```python
from build123d import *

# Parameters (mm, degrees)
EXTRUDE_1_DEPTH     = 3
SKETCH_3_R          = 7
CUT_EXTRUDE_1_DEPTH = 65.474801279
SKETCH_4_R          = 1
CUT_EXTRUDE_2_DEPTH = 65.474801279
FILLET_1_RADIUS     = 6
FILLET_1_LENGTH     = 3
EXTRUDE_2_DEPTH     = 2
SKETCH_7_R          = 4
CUT_EXTRUDE_3_DEPTH = 65.598761598
CUT_EXTRUDE_4_DEPTH = 2
SKETCH_9_R          = 0.537141257
CUT_EXTRUDE_5_DEPTH = 65.474801279
SKETCH_10_R         = 1.85
CUT_EXTRUDE_6_DEPTH = 1.5


with BuildPart() as part:
    # 草图1 → 凸台-拉伸1 (new body)
    with BuildSketch(Plane.XY):
        Polygon((-18, 0), (18, 0), (18, 5), (-12.599564267, 58), (-28, 58), (-28, 46), (-18, 46), align=None)
    extrude(amount=EXTRUDE_1_DEPTH)

    # 草图3 → 切除-拉伸1 (cut, through all)
    with BuildSketch(Plane.XY.offset(3)):
        with Locations((-6.476357534, 13.687539211)):
            Circle(SKETCH_3_R)
    extrude(amount=-CUT_EXTRUDE_1_DEPTH, mode=Mode.SUBTRACT)

    # 草图4 → 切除-拉伸2 (cut, through all)
    with BuildSketch(Plane.XY.offset(3)):
        with Locations((12, 2.5)):
            Circle(SKETCH_4_R)
        with Locations(Location((-12, 2.5, 0), (0, 0, 180))):
            Circle(SKETCH_4_R)
    extrude(amount=-CUT_EXTRUDE_2_DEPTH, mode=Mode.SUBTRACT)

    # 圆角1: full round fillet: the end face becomes a half cylinder, R = half its width
    fillet_1_face = Plane((-28, 52, 1.5), x_dir=(0, 0, 1), z_dir=(-1, 0, 0))  # on the end face: x along it, z out of the body
    fillet_1_slab = fillet_1_face.offset(-FILLET_1_RADIUS / 2) * Box(FILLET_1_LENGTH, 2 * FILLET_1_RADIUS, FILLET_1_RADIUS, mode=Mode.PRIVATE)  # the body's end, R deep
    fillet_1_round = Plane((-22, 52, 1.5), x_dir=(-1, 0, 0), z_dir=(0, 0, 1)) * Cylinder(FILLET_1_RADIUS, FILLET_1_LENGTH, mode=Mode.PRIVATE)  # its axis R under the face
    add(fillet_1_slab - fillet_1_round, mode=Mode.SUBTRACT)

    # 草图6 → 凸台-拉伸2 (add)
    with BuildSketch(Plane(origin=(0, 0, 0), x_dir=(-1, 0, 0), z_dir=(0, 0, -1))):
        with BuildLine():
            Line((22, 58), (12.599564267, 58))
            Line((12.599564267, 58), (7.650807626, 49.428502063))
            Line((7.650807626, 49.428502063), (7.650807626, 46))
            Line((7.650807626, 46), (22, 46))
            ThreePointArc((22, 46), (28, 52), (22, 58))
        make_face()
    extrude(amount=EXTRUDE_2_DEPTH)

    # 草图7 → 切除-拉伸3 (cut, through all)
    with BuildSketch(Plane.XY.offset(3)):
        with Locations((-22, 52)):
            Circle(SKETCH_7_R)
    extrude(amount=-CUT_EXTRUDE_3_DEPTH, mode=Mode.SUBTRACT)

    # 草图8 → 切除-拉伸4 (cut)
    with BuildSketch(Plane(origin=(0, 0, -2), x_dir=(-1, 0, 0), z_dir=(0, 0, -1))):
        Polygon((21.170465578, 55.913038799), (21.170465578, 48.086961201), (7.021339854, 49.472936706), (7.021339854, 54.618719507), align=None)
    extrude(amount=-CUT_EXTRUDE_4_DEPTH, mode=Mode.SUBTRACT)

    # 草图9 → 切除-拉伸5 (cut, through all)
    with BuildSketch(Plane(origin=(0, 0, 0), x_dir=(-1, 0, 0), z_dir=(0, 0, -1))):
        with Locations((16.5, 52)):
            Circle(SKETCH_9_R)
    extrude(amount=-CUT_EXTRUDE_5_DEPTH, mode=Mode.SUBTRACT)

    # 草图10 → 切除-拉伸6 (cut)
    with BuildSketch(Plane(origin=(0, 0, 0), x_dir=(-1, 0, 0), z_dir=(0, 0, -1))):
        with Locations((12, 2.5)):
            Circle(SKETCH_10_R)
        with Locations((-12, 2.5)):
            Circle(SKETCH_10_R)
    extrude(amount=-CUT_EXTRUDE_6_DEPTH, mode=Mode.SUBTRACT)


solid = part.part
```
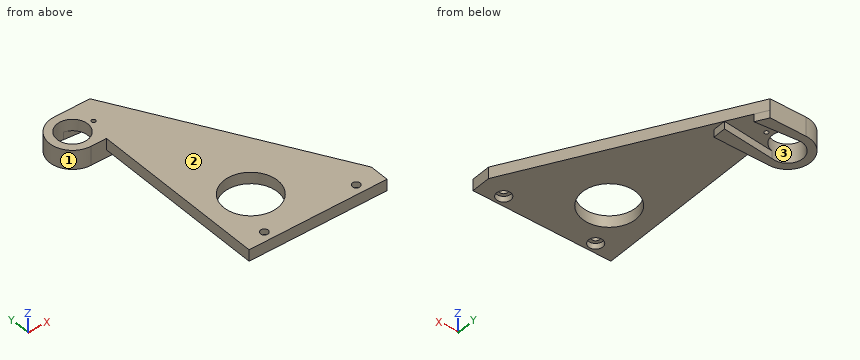
The model under review builds one solid part; all positions refer to its coordinate system, in mm. Face numbers are marked on the shaded views. Round coordinates to 2 decimals unless told otherwise and drop trailing zeros. Loops run counter-clockwise (first coordinate to the right, second up) from the corner with the lowest first, then second, coordinate; pieces in that order, holes last. Notation, with made-up numbers: M 45,51 L 91,51 A23 cw 91,75 Z; hole C 38,-40 d5. An arc over 180 degrees is marked long. Write item = value, one per line.
Item 1: For line 1 (X direction, y = 52, z = 1.4); line 2 (Y direction, x = -22, z = -0.4); line 3 (Y direction, x = -12, z = 0.85), list the stretches that pass through material, from the lowest coordinate up. Write a range as [from, to].
Return value:
line_1 = [-28, -26], [-18, -17.04], [-15.96, -9.14]
line_2 = [46, 48], [56, 58]
line_3 = [0, 0.65], [4.35, 9.39], [17.99, 56.96]
Item 2: Take a section at D-D on y = 25.5. Write out the cut boundary in (x, z).
Return value:
outline = M -18,0 L 6.16,0 L 6.16,3 L -18,3 Z
Item 3: Take a section at A-A on x = -19.5. Write out the cut boundary in (y, z), then the cut area to 3 significant figures.
Return value:
outline = M 46,-2 L 48.25,-2 L 48.25,0 L 48.88,0 L 48.88,3 L 46,3 Z; M 55.12,0 L 55.76,0 L 55.76,-2 L 58,-2 L 58,3 L 55.12,3 Z
area = 26.2 mm2
Item 4: Take a section at B-B on y = 14.5. Write out the cut boundary in (x, z).
Return value:
outline = M -18,0 L -13.43,0 L -13.43,3 L -18,3 Z; M 0.48,0 L 12.52,0 L 12.52,3 L 0.48,3 Z
Item 5: Take a section at C-C on x = 12. Write out the cut boundary in (y, z), then the cut area to 3 significant figures.
Return value:
outline = M 0,0 L 0.65,0 L 0.65,1.5 L 1.5,1.5 L 1.5,3 L 0,3 Z; M 3.5,1.5 L 4.35,1.5 L 4.35,0 L 15.39,0 L 15.39,3 L 3.5,3 Z
area = 37.6 mm2
Item 6: Insertion check: P1, Ø1.2, axis at x = -12, y = 2.5, coming from the +Z side; P2, Ø1, axis at y = 16.5, z = 1, coming from the -X side; P3, Ø3, axis at x = 4.5, z = 1.5, coming from the +Y side; P4, Ø1.1, axis at x = 13, y = 2, coming from the -Z side. Each pin has a flat end and moves straight along its axis. Give the tip position at first contact, or say it passes through.
Return value:
P1 = through
P2 = -18
P3 = 30.98
P4 = 1.5
Item 7: The part is to be moulded in two halves that separate along Y. For the marked faces 1, 2 and 3, say which applies: released by +Y, released by -Y, zero draft, split by the parting line, or undercut.
Return value:
face_1 = split by the parting line
face_2 = zero draft
face_3 = undercut
